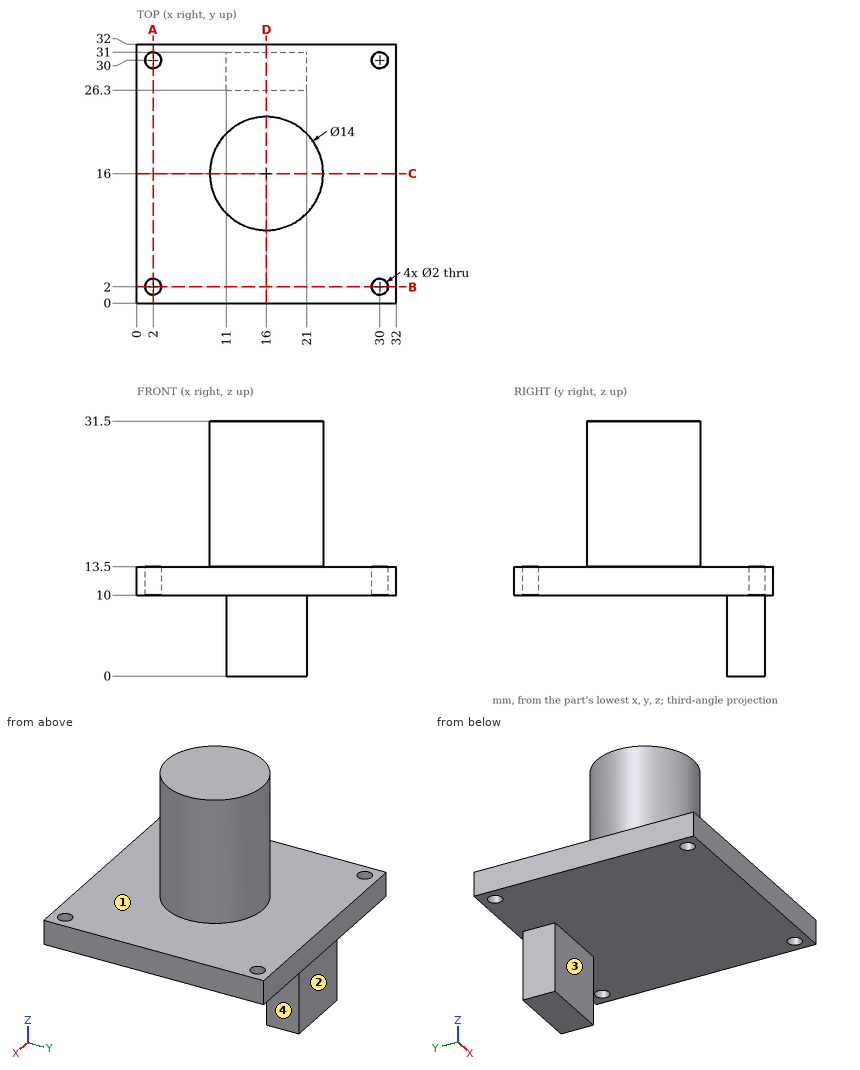
Source: three-view drawing plus pictorial views. Frame: mm from the lowest corner of the part. A direction names the side the tool comes from. Coordinates: 2 decimals unless noted, no trailing zeros. Loops run counter-clockwise (first coordinate to the right, second up) from the corner with the lowest first, then second, coordinate; pieces in that order, holes last. Notation, with made-up numbers: (59.25, -10) -> (118.25, -10) arc R27 cw to (118.25, 8) -> close; hole circle Ø1 at (-18, 42.25). An arc over 180 degrees is marked (long way). One line per item, written item: value.
(1) Pin query (flat end, axial travel): pin 1 Ø10 at (x, y) = (4, 18.5) entering from +Z; pin 2 Ø5 at (x, z) = (16, 5.5) entering from +Y; pin 3 Ø3 at (y, z) = (20, 15.5) entering from +X. Return the tip coordinate at first contact, or that it passes through.
Answer below:
pin 1: stops at z = 13.5
pin 2: stops at y = 31
pin 3: stops at x = 22.54
(2) Cut plane C-C (y = 16). Output: boundary loops of the cut face in (x, z).
Answer below:
outline: (0, 10) -> (32, 10) -> (32, 13.5) -> (23, 13.5) -> (23, 31.5) -> (9, 31.5) -> (9, 13.5) -> (0, 13.5) -> close
(3) Cut plane D-D (x = 16). Output: boundary loops of the cut face in (y, z).
Answer below:
outline: (0, 10) -> (26.3, 10) -> (26.3, 0) -> (31, 0) -> (31, 10) -> (32, 10) -> (32, 13.5) -> (23, 13.5) -> (23, 31.5) -> (9, 31.5) -> (9, 13.5) -> (0, 13.5) -> close
(4) Set-up query: the marked faces 1, 2, 3 and 4. Return all of +Z, -Z, +X, -X, +Y, -Y with unobstructed straight access to the full face (end or side cutting, diameter ignored); none if empty.
Answer below:
face 1: +Z
face 2: -Z, +X, -X, +Y
face 3: -Z, +X, -X, -Y
face 4: -Z, +X, +Y, -Y
(5) Ray query, line 1 along Y through (x, z) = (30, 12.2); line 2 along Z through (x, y) = (19, 15.5). Return the intervals inside material, ascending.
Answer below:
line 1: y = 0 to 1, 3 to 29, 31 to 32
line 2: z = 10 to 31.5
(6) Cut plane A-A (x = 2). Output: boundary loops of the cut face in (y, z), then the cut area to 3 significant figures.
Answer below:
outline: (0, 10) -> (1, 10) -> (1, 13.5) -> (0, 13.5) -> close; (3, 10) -> (29, 10) -> (29, 13.5) -> (3, 13.5) -> close; (31, 10) -> (32, 10) -> (32, 13.5) -> (31, 13.5) -> close
area: 98.0 mm2
